Here's how the part is built. I have some questions about the finished solid (model axes, mm). A direction names the side the tool comes from. Coordinates: 2 decimals unless noted, no trailing zeros. Write each loop counter-clockwise with the first axis right and the second up, starting at its lowest first coordinate (ties: lowest second). Pieces come first, ordered by that corner, then holes. Notation, with made-up numbers: (-31.75, 48.25) -> (-11.75, 48.25) arc R17 ccw to (-11.75, 71.25) -> close; hole circle Ø6 at (-40, 74). An arc over 180 degrees is marked (long way). Use a Markdown table: item, result. Add a question column.
Item 1: If I drill on line 1 along Y through (x, z) = (0, 17); line 2 along X through (y, z) = (2.5, 24); line 3 along Y through (x, z) = (-15, 21.75), over which ranges is the centre line in solid material (lowest first)? Write a range as from..to.
Item 2: On a 3-axis mill with a long thin cutter (end or side, diameter ignored), from which of +Z, -Z, +X, -X, +Y, -Y can I reach the whole of each face in a straight line? I mean faces 4 (the cylindrical face through (-5.85, -26.36, 14.79)), 5 (the flat face through (-34, -33, 10)). Say none if no direction works.
Item 3: Imagine slicing it at A-A, the plane x = 0. Write out the boundary of the cut face in (y, z).
Item 4: Imagine slicing it at D-D, the plane y = -38. Write out the boundary of the cut face in (x, z).
Item 5: Imagine slicing it at B-B, the plane z = 12.25. Write out the boundary of the cut face in (x, y).
Item 6: If we mould it in two halves opening along X, with no side actions, what happens to faces 1 (the flat face through (-35, 0, 10)), 2 (the cylindrical face through (-11.923, -53.692, 14.79)), 3 (the flat face through (-13, -24, 0))? For each: pulls with the +X half, pulls with the -X half, needs draft (parallel to the pull), parting line crosses it, or undercut.
Item 7: Will these pins go through, and if not, where does the flat tip stop? pin 1 Ø15 at (x, y) = (-34.5, 0) entering from +Z; pin 2 Ø1 at (x, z) = (6.5, 21) entering from -Y; pin 3 Ø8 at (y, z) = (14.5, 14) entering from -X; pin 4 Ø1 at (y, z) = (6.5, 26) entering from -X.
Item 8: Imagine slicing it at C-C, the plane y = 0. Write out the boundary of the cut face in (x, z).
```python
from build123d import *

# Parameters (mm, degrees)
SKETCH1_R           = 55
SKETCH1_R_2         = 27
BOSS_EXTRUDE1_DEPTH = 10
SKETCH2_R           = 55
SKETCH2_R_2         = 50
SKETCH2_R_3         = 47
SKETCH2_R_4         = 4.75
SKETCH2_R_5         = 27
BOSS_EXTRUDE4_DEPTH = 20


with BuildPart() as part:
    # Sketch1 → Boss-Extrude1 (new body)
    with BuildSketch(Plane.XY):
        Circle(SKETCH1_R)
        Circle(SKETCH1_R_2, mode=Mode.SUBTRACT)
    extrude(amount=BOSS_EXTRUDE1_DEPTH)

    # Sketch2 → Boss-Extrude4 (add)
    # profile 1 of 2: a face of its own
    with BuildSketch(Plane.XY.offset(10)):
        Circle(SKETCH2_R)
        Circle(SKETCH2_R_2, mode=Mode.SUBTRACT)
    # profile 2 of 2: a face of its own
    with BuildSketch(Plane.XY.offset(10)):
        Circle(SKETCH2_R_3)
        with Locations((-34.5, 0)):
            Circle(SKETCH2_R_4, mode=Mode.SUBTRACT)
        with Locations((34.5, 0)):
            Circle(SKETCH2_R_4, mode=Mode.SUBTRACT)
        Circle(SKETCH2_R_5, mode=Mode.SUBTRACT)
    extrude(amount=BOSS_EXTRUDE4_DEPTH)


solid = part.part
```
Ans:
| question | item | result |
|---|---|---|
| 1 | line 1 | y = -55..-50, -47..-27, 27..47, 50..55 |
| 1 | line 2 | x = -54.94..-49.94, -46.93..-38.54, -30.46..-26.88, 26.88..30.46, 38.54..46.93, 49.94..54.94 |
| 1 | line 3 | y = -52.92..-47.7, -44.54..-22.45, 22.45..44.54, 47.7..52.92 |
| 2 | face 4 | +Z, -Z |
| 2 | face 5 | +Z |
| 3 | outline | (-55, 0) -> (-27, 0) -> (-27, 30) -> (-47, 30) -> (-47, 10) -> (-50, 10) -> (-50, 30) -> (-55, 30) -> close; (27, 0) -> (55, 0) -> (55, 30) -> (50, 30) -> (50, 10) -> (47, 10) -> (47, 30) -> (27, 30) -> close |
| 4 | outline | (-39.76, 0) -> (39.76, 0) -> (39.76, 30) -> (32.5, 30) -> (32.5, 10) -> (27.66, 10) -> (27.66, 30) -> (-27.66, 30) -> (-27.66, 10) -> (-32.5, 10) -> (-32.5, 30) -> (-39.76, 30) -> close |
| 5 | outline | circle Ø110 at (0, 0); circle Ø94 at (0, 0); hole circle Ø100 at (0, 0); hole circle Ø9.5 at (-34.5, 0); hole circle Ø54 at (0, 0); hole circle Ø9.5 at (34.5, 0) |
| 6 | face 1 | undercut |
| 6 | face 2 | parting line crosses it |
| 6 | face 3 | needs draft |
| 7 | pin 1 | stops at z = 30 |
| 7 | pin 2 | stops at y = -54.67 |
| 7 | pin 3 | stops at x = -53.99 |
| 7 | pin 4 | stops at x = -54.67 |
| 8 | outline | (-55, 0) -> (-27, 0) -> (-27, 30) -> (-29.75, 30) -> (-29.75, 10) -> (-39.25, 10) -> (-39.25, 30) -> (-47, 30) -> (-47, 10) -> (-50, 10) -> (-50, 30) -> (-55, 30) -> close; (27, 0) -> (55, 0) -> (55, 30) -> (50, 30) -> (50, 10) -> (47, 10) -> (47, 30) -> (39.25, 30) -> (39.25, 10) -> (29.75, 10) -> (29.75, 30) -> (27, 30) -> close |
